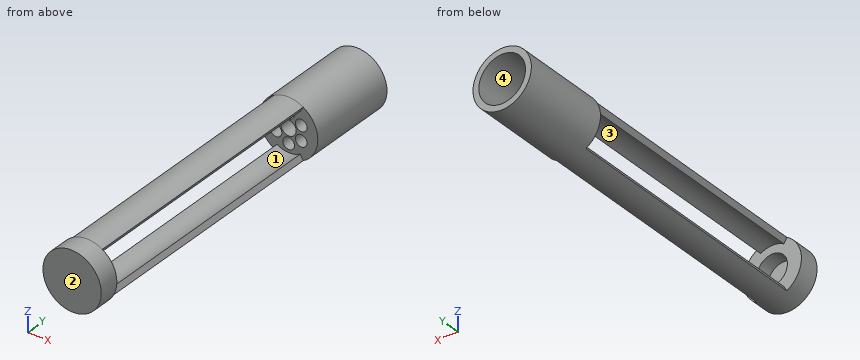
```python
from build123d import *

# Parameters (mm, degrees)
SKETCH1_R            = 5
BOSS_EXTRUDE1_DEPTH  = 3.5
SKETCH2_R            = 2.6
CUT_EXTRUDE1_DEPTH   = 2.5
BOSS_EXTRUDE2_DEPTH  = 45
SKETCH14_R           = 5
SKETCH14_R_2         = 1.3
BOSS_EXTRUDE8_DEPTH  = 3
SKETCH15_R           = 5
SKETCH15_R_2         = 2.6
BOSS_EXTRUDE9_DEPTH  = 2.5
SKETCH7_R            = 1
CUT_EXTRUDE2_DEPTH   = 2
CIRPATTERN1_COUNT    = 6
CUT_EXTRUDE3_START   = -3.5
SKETCH12_R           = 0.2
CUT_EXTRUDE3_DEPTH   = 4.5
CIRPATTERN2_COUNT    = 6
SKETCH16_R           = 5
SKETCH16_R_2         = 4
BOSS_EXTRUDE10_DEPTH = 10


with BuildPart() as part:
    # Sketch1 → Boss-Extrude1 (new body)
    with BuildSketch(Plane(origin=(0, 0, 0), x_dir=(1, 0, 0), z_dir=(0, 1, 0))):
        Circle(SKETCH1_R)
    extrude(amount=BOSS_EXTRUDE1_DEPTH)

    # Sketch2 → Cut-Extrude1 (cut)
    with BuildSketch(Plane(origin=(0, 3.5, 0), x_dir=(1, 0, 0), z_dir=(0, 1, 0))):
        Circle(SKETCH2_R)
    extrude(amount=-CUT_EXTRUDE1_DEPTH, mode=Mode.SUBTRACT)

    # Sketch3 → Boss-Extrude2 (add)
    with BuildSketch(Plane(origin=(0, 3.5, 0), x_dir=(1, 0, 0), z_dir=(0, 1, 0))):
        with BuildLine():
            ThreePointArc((-2.5, -4.330127019), (0, -5), (2.5, -4.330127019))
            Line((2.5, -4.330127019), (2, -3.464101615))
            ThreePointArc((2, -3.464101615), (0, -4), (-2, -3.464101615))
            Line((-2, -3.464101615), (-2.5, -4.330127019))
        make_face()
        with BuildLine():
            ThreePointArc((2.5, 4.330127019), (0, 5), (-2.5, 4.330127019))
            Line((-2.5, 4.330127019), (-2, 3.464101615))
            ThreePointArc((-2, 3.464101615), (0, 4), (2, 3.464101615))
            Line((2, 3.464101615), (2.5, 4.330127019))
        make_face()
    extrude(amount=BOSS_EXTRUDE2_DEPTH)

    # Sketch14 → Boss-Extrude8 (add)
    with BuildSketch(Plane(origin=(0, 48.5, 0), x_dir=(1, 0, 0), z_dir=(0, 1, 0))):
        Circle(SKETCH14_R)
        Circle(SKETCH14_R_2, mode=Mode.SUBTRACT)
    extrude(amount=BOSS_EXTRUDE8_DEPTH)

    # Sketch15 → Boss-Extrude9 (add)
    with BuildSketch(Plane(origin=(0, 51.5, 0), x_dir=(1, 0, 0), z_dir=(0, 1, 0))):
        Circle(SKETCH15_R)
        Circle(SKETCH15_R_2, mode=Mode.SUBTRACT)
    extrude(amount=BOSS_EXTRUDE9_DEPTH)

    # Sketch7 → Cut-Extrude2 (cut)
    with BuildSketch(Plane.XZ.offset(-48.5)):
        with Locations((0, 2.5)):
            Circle(SKETCH7_R)
    cut_extrude2 = extrude(amount=-CUT_EXTRUDE2_DEPTH, mode=Mode.SUBTRACT)

    # CirPattern1: Cut-Extrude2 ×6 about axis
    cirpattern1_axis = Axis((0, 0, 0), (0, 1, 0))
    for i in range(1, CIRPATTERN1_COUNT):
        add(cut_extrude2.rotate(cirpattern1_axis, i * 360 / CIRPATTERN1_COUNT), mode=Mode.SUBTRACT)

    # Sketch12 → Cut-Extrude3 (cut)
    with BuildSketch(Plane(origin=(0, 54, 0), x_dir=(1, 0, 0), z_dir=(0, 1, 0)).offset(CUT_EXTRUDE3_START)):
        with Locations((0, -3)):
            Circle(SKETCH12_R)
    cut_extrude3 = extrude(amount=CUT_EXTRUDE3_DEPTH, mode=Mode.SUBTRACT)

    # CirPattern2: Cut-Extrude3 ×6 about axis
    cirpattern2_axis = Axis((0, 0, 0), (0, 1, 0))
    for i in range(1, CIRPATTERN2_COUNT):
        add(cut_extrude3.rotate(cirpattern2_axis, i * 360 / CIRPATTERN2_COUNT), mode=Mode.SUBTRACT)

    # Sketch16 → Boss-Extrude10 (add)
    with BuildSketch(Plane(origin=(0, 54, 0), x_dir=(1, 0, 0), z_dir=(0, 1, 0))):
        Circle(SKETCH16_R)
        Circle(SKETCH16_R_2, mode=Mode.SUBTRACT)
    extrude(amount=BOSS_EXTRUDE10_DEPTH)


solid = part.part
```
Verification items for the finished model (mm, model axes). Face numbers are marked on the shaded views. A direction names the side the tool comes from. Round coordinates to 2 decimals unless told otherwise and drop trailing zeros. Write each loop counter-clockwise with the first axis right and the second up, starting at its lowest first coordinate (ties: lowest second). Pieces come first, ordered by that corner, then holes. Notation, with made-up numbers: (44, 83) -> (73, 83) arc R20 cw to (73, 113) -> close; hole circle Ø1 at (49.25, 48.5). An arc over 180 degrees is marked (long way). Write each question's results on one line, items separated by ' | '.
Q1. Sectioned sample at B-B, the plane y = 55. Record the boundary of the cut face in (x, z).
Derived:
outline: circle Ø10 at (0, 0); hole circle Ø8 at (0, 0)
Q2. Thickness scan on probe 1 along Z at (x, y) = (0, 52.2); probe 2 along Y at (x, z) = (-2.75, 2.25); probe 3 along X at (y, z) = (50.2, 0). Record the ranges inside material, lowest first.
Derived:
probe 1: z = -5 to -3.2, -2.8 to -2.6, 2.6 to 2.8, 3.2 to 5 | probe 2: y = 0 to 3.5, 48.5 to 54 | probe 3: x = -5 to -1.3, 1.3 to 5
Q3. Access from +Z, -Z, +X, -X, +Y, -Y to the whole of each face (thin tool, end or side, straight path). Record for the marked faces 3 and 4.
Derived:
face 3: none | face 4: +Y
Q4. Sectioned sample at A-A, the plane y = 34.5. Record the boundary of the cut face in (x, z), and give its area (3 significant figures).
Derived:
outline: (-2.5, -4.33) arc R5 ccw to (2.5, -4.33) -> (2, -3.46) arc R4 cw to (-2, -3.46) -> close; (-2.5, 4.33) -> (-2, 3.46) arc R4 cw to (2, 3.46) -> (2.5, 4.33) arc R5 ccw to start | area: 9.42 mm²
Q5. Draft check along X on the marked faces 1 and 2. Enter one of: released by +X, released by -X, zero draft, split by the parting line, or undercut.
Derived:
face 1: undercut | face 2: zero draft
Q6. Go/stop test with flat-tipped pins: pin 1 Ø1.2 at (x, z) = (0, 2.5) entering from +Y; pin 2 Ø1 at (y, z) = (52.5, -3) entering from +X; pin 3 Ø2 at (y, z) = (27, 4) entering from -X. Record where each tip stops, or that it passes through.
Derived:
pin 1: stops at y = 54 | pin 2: stops at x = 4.33 | pin 3: stops at x = -2.5
